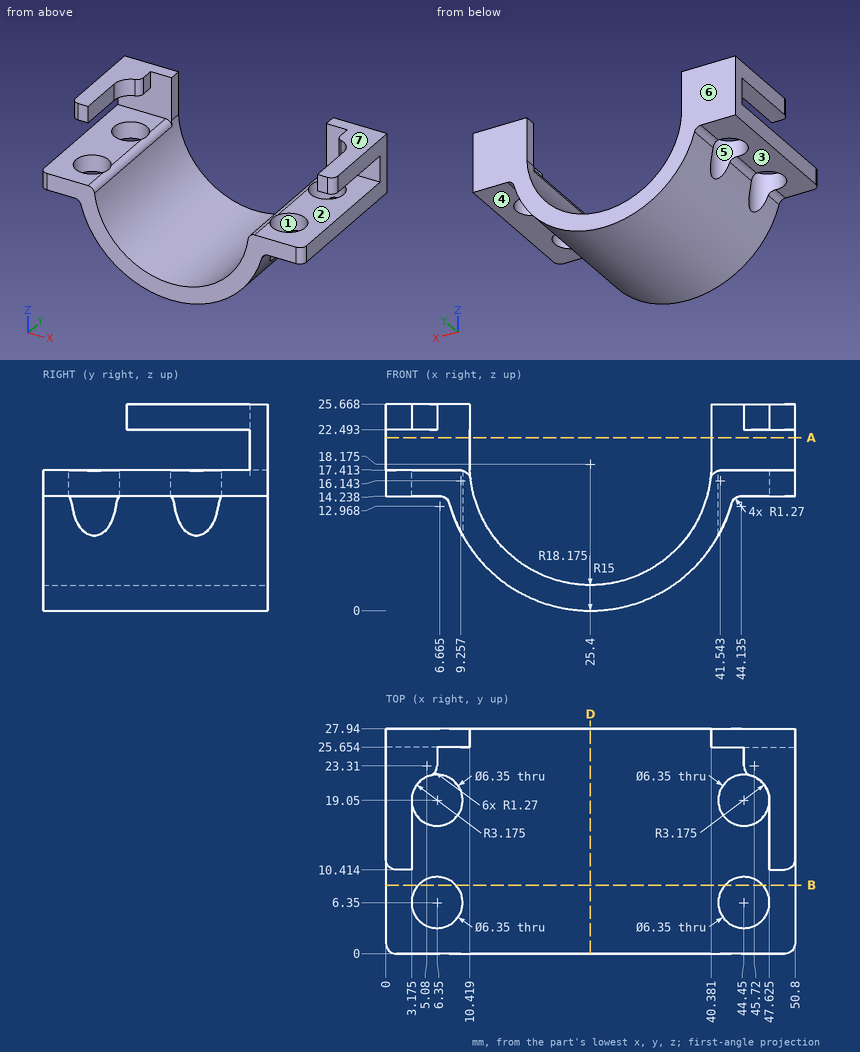
Job drawing, mm, ordinate dimensions from the low corner. One solid piece. A direction names the side the tool comes from. Give positions to 0.01 mm unless a question says otherwise; leave off trailing zeros. Order: outer loops, then holes, each group sorted by start corner. A loop starts at its lowest first (then second) coordinate and runs counter-clockwise, first axis right, second up. Notation, with made-up numbers: (-19.75, 48) - (-15.75, 48) arc R11 cw to (-15.75, 57) - close; hole circle Ø4 at (-2, 46). An arc over 180 degrees is marked (long way). Return JSON: item names as keys, results as strings.
1) Probe line 1 (Y direction, x = 45.5, z = 14.75); line 2 (Z direction, x = 2, y = 24.25); line 3 (X direction, y = 20.75, z = 24.5). List the from-to ranges inside material, lowest first. Write a range as from..to.
Geometry says:
{"line 1": "0..3.35, 9.35..16.05, 22.05..27.94", "line 2": "14.24..17.41, 22.49..25.67", "line 3": "0..3.67, 47.13..50.8"}
2) Cut at B-B, the plane y = 8.5. Count the separate pieces of the cut face and the enclosed holes in it, plus the area to 3 significant figures.
Geometry says:
{"separate pieces": "3", "enclosed holes": "0", "area": "174 mm²"}
3) 3-axis set-ups, long thin cutter, end or side, ignore diameter. For the marked faces 1, 2, 3 and 4: which of +Z, -Z, +X, -X, +Y, -Y reach the whole face in a straight line?
Geometry says:
{"face 1": "+Z, -Z", "face 2": "+X, -X, -Y", "face 3": "-Z, -X, +Y, -Y", "face 4": "-Z, +X, +Y, -Y"}
4) Pull direction Y, two halves, no side cores. Call the marked faces 5, 6 and 7: pulls with the +Y half, pulls with the -Y half, needs draft (parallel to the pull), parting line crosses it, or undercut.
Geometry says:
{"face 5": "undercut", "face 6": "pulls with the +Y half", "face 7": "needs draft"}
5) Cut at A-A, the plane z = 21.5. Give the cut face in (x, y).
Geometry says:
{"outline": "(0, 25.65) - (10.42, 25.65) - (10.42, 27.94) - (0, 27.94) - close; (40.38, 25.65) - (50.8, 25.65) - (50.8, 27.94) - (40.38, 27.94) - close"}
6) Flat gauge pins, fed straight in: P1, Ø10, axis at x = 42, z = 6, coming from the +Y side; P2, Ø4.5, axis at x = 6, y = 17.5, coming from the +Z side; P3, Ø3.5, axis at x = 2.5, y = 14.5, coming from the -Z side; P4, Ø3, axis at y = 22, z = 9.5, coming from the +X side. Where does each tip first touch, or does it go through?
Geometry says:
{"P1": "y = 27.94", "P2": "z = 17.41", "P3": "z = 14.24", "P4": "x = 42.1"}
7) Cut at D-D, the plane x = 25.4. Give the cut face in (y, z) (1 decimal).
Geometry says:
{"outline": "(0, 0) - (27.9, 0) - (27.9, 3.2) - (0, 3.2) - close"}
